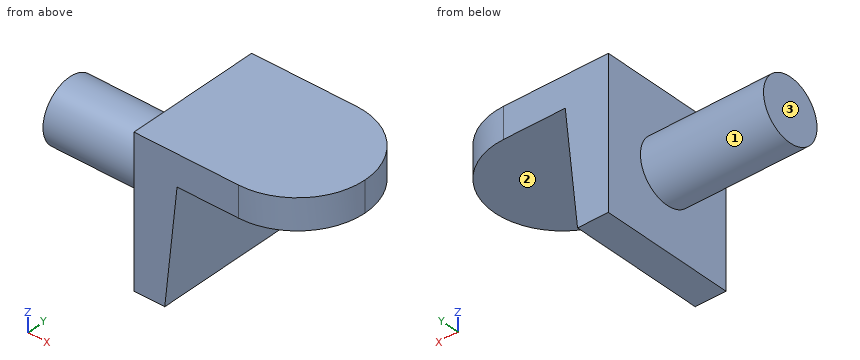
from build123d import *

# Parameters (mm, degrees)
F1_DEPTH = 11
F4_DEPTH = 12.001
F5_R     = 2.5
F6_DEPTH = 10


with BuildPart() as f1:
    # F0 (on Front) → F1 (new body)
    with BuildSketch(Plane.XZ):
        Polygon((14, 0), (0, 0), (0, -12), (2.5, -12), (3.5, -2.5), (14, -2.5), align=None)
    extrude(amount=F1_DEPTH)


with BuildPart() as f1_1:
    # F2: moved
    add(f1.part.moved(Location((0, 5.5, 0))))

    # F3 (on face) → F4 (cut, through all)
    with BuildSketch(Plane.XY):
        with BuildLine():
            ThreePointArc((8.5, 5.5), (12.3890872965, 3.8890872965), (14, 0))
            Line((14, 0), (14, 5.5))
            Line((14, 5.5), (8.5, 5.5))
        make_face()
        with BuildLine():
            ThreePointArc((14, 0), (12.3890872965, -3.8890872965), (8.5, -5.5))
            Line((8.5, -5.5), (14, -5.5))
            Line((14, -5.5), (14, 0))
        make_face()
    extrude(amount=-F4_DEPTH, mode=Mode.SUBTRACT)

    # F5 (on face) → F6 (join)
    with BuildSketch(Plane(origin=(0, 0, 0), x_dir=(0, -1, 0), z_dir=(-1, 0, 0))):
        with Locations((0, -6)):
            Circle(F5_R)
    extrude(amount=F6_DEPTH)


solid = f1_1.part
Read the model definition and answer for the solid it produces. Units are mm, in the model's axes. Face numbers are marked on the shaded views. A direction names the side the tool comes from. Round coordinates to 2 decimals unless told otherwise and drop trailing zeros. Order: outer loops, then holes, each group sorted by start corner. A loop starts at its lowest first (then second) coordinate and runs counter-clockwise, first axis right, second up.
1) The part is cut by section D-D on y = 1. Write down the section's boundary in (x, z), plus the area to 3 significant figures.
2) The part is cut by section A-A on y = -1.75. Write down the section's boundary in (x, z), plus the area to 3 significant figures.
3) Flat-ended cylindrical pins translate along their axes: pin 1 (6 mm diameter, centred on y = -3.5, z = -4, fed in from +X); pin 2 (4 mm diameter, centred on x = 11, z = -4, fed in from +Y); pin 3 (4 mm diameter, centred on x = -6.5, z = -3.5, fed in from -Y). Find the tip coordinate at first contact, or state that the pin passes through.
4) For the marked faces 1, 2 and 3, determine the directions among +Z, -Z, +X, -X, +Y, -Y from which every point of the face is accessible in a straight line to the end or side of a thin tool.
5) The part is cut by section C-C on z = -6. Write down the section's boundary in (x, y), plus the area to 3 significant figures.
6) The part is cut by section B-B on x = 5.5. Write down the section's boundary in (y, z), plus the area to 3 significant figures.
7) Straight lines are drawn through the part: L1, parallel to Z at x = 5, y = 1.25; L2, parallel to X at y = -1.5, z = -2.75; L3, parallel to Z at x = -4.5, y = 1. For each, find the intervals that lie inside material, in ascending order.
Resolved:
1. outline: (-10, -8.29) - (0, -8.29) - (0, -12) - (2.5, -12) - (3.5, -2.5) - (13.91, -2.5) - (13.91, 0) - (0, 0) - (0, -3.71) - (-10, -3.71) - close
1. area: 109 mm2
2. outline: (-10, -7.79) - (0, -7.79) - (0, -12) - (2.5, -12) - (3.5, -2.5) - (13.71, -2.5) - (13.71, 0) - (0, 0) - (0, -4.21) - (-10, -4.21) - close
2. area: 98.5 mm2
3. pin 1: stops at x = 13.93
3. pin 2: stops at y = 5.37
3. pin 3: stops at y = -2.45
4. face 1: -X
4. face 2: -Z, +X, +Y, -Y
4. face 3: +Z, -Z, -X, +Y, -Y
5. outline: (-10, -2.5) - (0, -2.5) - (0, -5.5) - (3.13, -5.5) - (3.13, 5.5) - (0, 5.5) - (0, 2.5) - (-10, 2.5) - close
5. area: 84.4 mm2
6. outline: (-5.5, -2.5) - (5.5, -2.5) - (5.5, 0) - (-5.5, 0) - close
6. area: 27.5 mm2
7. L1: z = -2.5 to 0
7. L2: x = 0 to 3.47
7. L3: z = -8.29 to -3.71
